Autodesk Inventor part; units mm, degrees
ref_plane "YZ Plane" through (0, 0, 0) normal (1, 0, 0) x (0, 1, 0)
ref_plane "XZ Plane" through (0, 0, 0) normal (0, 1, 0) x (-1, 0, 0)
ref_plane "XY Plane" through (0, 0, 0) normal (0, 0, 1) x (1, 0, 0)
sketch "Эскиз1" plane through (0, 0, 0) normal (0, 1, 0) x (-1, 0, 0)
  line L0 (0, 0) -> (-85, 0)
  line L1 (-85, 0) -> (-85, 150)
  line L2 (-85, 150) -> (0, 150)
  line L3 (0, 150) -> (0, 0)
  dimension "d0" = 85
  dimension "d1" = 150
extrude "Выдавливание1" add sketch "Эскиз1" along normal blind 50
sketch "Эскиз2" plane through (0, 50, 0) normal (0, 1, 0) x (1, 0, 0)
  line L0 (0, 0) -> (0, -150)
  line L1 (0, 0) -> (42.5, 0)
  line L2 (85, 0) -> (0, 0)
  line L3 (42.5, 0) -> (42.5, -28)
  dimension "d5" = 42.5
  dimension "d6" = 28
hole "Отверстие1" at (42.5, 50, 28) direction (0, -1, 0) diameter 8 end through all
sketch "Эскиз3" plane through (0, 50, 0) normal (0, 1, 0) x (1, 0, 0)
  line L0 (0, 0) -> (0, -150)
  line L1 (0, 0) -> (0, -120)
  line L2 (0, -120) -> (42.5, -120)
  circle A0 centre (42.5, -120) radius 5
  dimension "d14" = 120
  dimension "d15" = 42.5
  dimension "d16" = 10
extrude "Выдавливание2" add sketch "Эскиз3" along normal blind 70
fillet "Сопряжение2" radius 7.5 4 edges at (0, 25, 0) (85, 25, 0) (85, 25, 150) (0, 25, 150)
properties part number "РедукторСмещенный"
Geometry: final body of the model. Coordinates: model frame, mm. Round coordinates to 2 decimals unless told otherwise and drop trailing zeros. Write each loop counter-clockwise with the first axis right and the second up, starting at its lowest first coordinate (ties: lowest second). Pieces come first, ordered by that corner, then holes. Notation, with made-up numbers: (-9.5, 11) -> (-5.5, 11) arc R18 cw to (-5.5, 32) -> close; hole circle Ø11 at (74, 1.5). An arc over 180 degrees is marked (long way). Return JSON: item names as keys, results as strings.
Q1. Ray query, line 1 (X direction, y = 21, z = 28); line 2 (Z direction, x = 42.5, y = 13.5); line 3 (X direction, y = 42.5, z = 7). Return the intervals inside material, ascending.
From the geometry:
{"line 1": "0 to 38.5, 46.5 to 85", "line 2": "0 to 24, 32 to 150", "line 3": "0.02 to 84.98"}
Q2. Section C-C on z = 120. Return the cut outline in (x, y), and give its area (3 significant figures).
From the geometry:
{"outline": "(0, 0) -> (85, 0) -> (85, 50) -> (47.5, 50) -> (47.5, 120) -> (37.5, 120) -> (37.5, 50) -> (0, 50) -> close", "area": "4,950 mm2"}
Q3. Section A-A on x = 42.5. Return the cut outline in (y, z), and give its area (3 significant figures).
From the geometry:
{"outline": "(0, 0) -> (50, 0) -> (50, 24) -> (0, 24) -> close; (0, 32) -> (50, 32) -> (50, 115) -> (120, 115) -> (120, 125) -> (50, 125) -> (50, 150) -> (0, 150) -> close", "area": "7,800 mm2"}
Q4. Section D-D on y = 90.5. Return the cut outline in (x, z).
From the geometry:
{"outline": "circle Ø10 at (42.5, 120)"}
Q5. Mould query, pull axis X, two halves, no side actions, for faces 1 (the flat face through (0, 25, 76)), 2 (the cylindrical face through (37.505, 84.51, 120.22)), 3 (the cylindrical face through (38.534, 24.65, 27.479)). Classes: +X half, -X half, draft (parallel to the pull), parting line (faces both ways), or undercut.
From the geometry:
{"face 1": "-X half", "face 2": "parting line", "face 3": "undercut"}
Q6. Section B-B on z = 28. Return the cut outline in (x, y), and give its area (3 significant figures).
From the geometry:
{"outline": "(0, 0) -> (38.5, 0) -> (38.5, 50) -> (0, 50) -> close; (46.5, 0) -> (85, 0) -> (85, 50) -> (46.5, 50) -> close", "area": "3,850 mm2"}
Q7. First-contact query: pin 1 Ø5 at (x, z) = (42.5, 28) entering from -Y; pin 2 Ø4 at (x, z) = (26, 43.5) entering from -Y. Flat tips, straight axial feed; report the tip coordinate or a pass-through.
From the geometry:
{"pin 1": "through", "pin 2": "y = 0"}
